CAD build for the part. Positions are in the model's coordinates, mm. Face numbers are marked on the shaded views. A direction names the side the tool comes from. Coordinates: 2 decimals unless noted, no trailing zeros. Loops run counter-clockwise (first coordinate to the right, second up) from the corner with the lowest first, then second, coordinate; pieces in that order, holes last. Notation, with made-up numbers: (-5.5, 77) -> (7.5, 77) arc R11 cw to (7.5, 82) -> close; hole circle Ø11 at (-10, 31.5). An arc over 180 degrees is marked (long way). Answer as a JSON object with one key per item and string values. Group by question number.
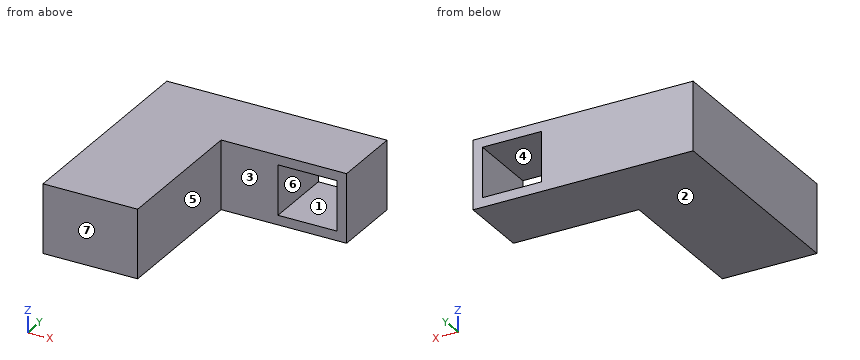
from build123d import *

# Parameters (mm, degrees)
SKETCH1_W           = 16.5
SKETCH1_H           = 14.5
SKETCH1_W_2         = 12.5
SKETCH1_H_2         = 10.5
BOSS_EXTRUDE1_DEPTH = 15
SKETCH2_W           = 14.5
SKETCH2_H           = 15
BOSS_EXTRUDE2_DEPTH = 30
SKETCH3_W           = 20
SKETCH3_H           = 14.5
BOSS_EXTRUDE3_DEPTH = 31


with BuildPart() as part:
    # Sketch1 → Boss-Extrude1 (new body)
    with BuildSketch(Plane(origin=(0, 0, 0), x_dir=(1, 0, 0), z_dir=(0, 1, 0))):
        with Locations((6.25, -5.25)):
            Rectangle(SKETCH1_W, SKETCH1_H)
        with Locations((6.25, -5.25)):
            Rectangle(SKETCH1_W_2, SKETCH1_H_2, mode=Mode.SUBTRACT)
    extrude(amount=BOSS_EXTRUDE1_DEPTH)

    # Sketch2 → Boss-Extrude2 (add)
    with BuildSketch(Plane.ZY.offset(2)):
        with Locations((5.25, 7.5)):
            Rectangle(SKETCH2_W, SKETCH2_H)
    extrude(amount=BOSS_EXTRUDE2_DEPTH)

    # Sketch3 → Boss-Extrude3 (add)
    with BuildSketch(Plane(origin=(0, 0, 0), x_dir=(-1, 0, 0), z_dir=(0, -1, 0))):
        with Locations((22, -5.25)):
            Rectangle(SKETCH3_W, SKETCH3_H)
    extrude(amount=BOSS_EXTRUDE3_DEPTH)


solid = part.part
Item 1: Drill centre lines: L1, parallel to X at y = 11, z = 2.5; L2, parallel to X at y = -13.5, z = 11; L3, parallel to Y at x = -5, z = 4. Where is each one in solid material? Low to high.
Item 2: Band-saw the part on D-D, the plane y = -19. List the corners of the cut face in (x, z), and give its area (3 significant figures).
Item 3: Band-saw the part on B-B, the plane y = 7. List the corners of the cut face in (x, z), and give its area (3 significant figures).
Item 4: 3-axis set-ups, long thin cutter, end or side, ignore diameter. For the marked faces 5, 6 and 7: which of +Z, -Z, +X, -X, +Y, -Y reach the whole face in a straight line?
Item 5: Band-saw the part on C-C, the plane x = 1.5. List the corners of the cut face in (y, z), and give its area (3 significant figures).
Item 6: Pull direction Z, two halves, no side cores. Call the marked faces 1, 2, 3 and 4: +Z half, -Z half, draft (parallel to the pull), parting line (faces both ways), or undercut.
Item 7: Band-saw the part on A-A, the plane z = 2.5. List the corners of the cut face in (x, y), and give its area (3 significant figures).
Reply:
{
 "1": {"L1": "-32 to 0, 12.5 to 14.5", "L2": "-32 to -12", "L3": "0 to 15"},
 "2": {"outline": "(-32, -2) -> (-12, -2) -> (-12, 12.5) -> (-32, 12.5) -> close", "area": "290 mm²"},
 "3": {"outline": "(-32, -2) -> (14.5, -2) -> (14.5, 12.5) -> (-32, 12.5) -> close; hole (0, 0) -> (12.5, 0) -> (12.5, 10.5) -> (0, 10.5) -> close", "area": "543 mm²"},
 "4": {"face 5": "+Z, -Z, +X, -Y", "face 6": "+Y, -Y", "face 7": "+Z, -Z, +X, -X, -Y"},
 "5": {"outline": "(0, -2) -> (15, -2) -> (15, 0) -> (0, 0) -> close; (0, 10.5) -> (15, 10.5) -> (15, 12.5) -> (0, 12.5) -> close", "area": "60.0 mm²"},
 "6": {"face 1": "undercut", "face 2": "-Z half", "face 3": "draft", "face 4": "undercut"},
 "7": {"outline": "(-32, -31) -> (-12, -31) -> (-12, 0) -> (0, 0) -> (0, 15) -> (-32, 15) -> close; (12.5, 0) -> (14.5, 0) -> (14.5, 15) -> (12.5, 15) -> close", "area": "1,130 mm²"}
}
